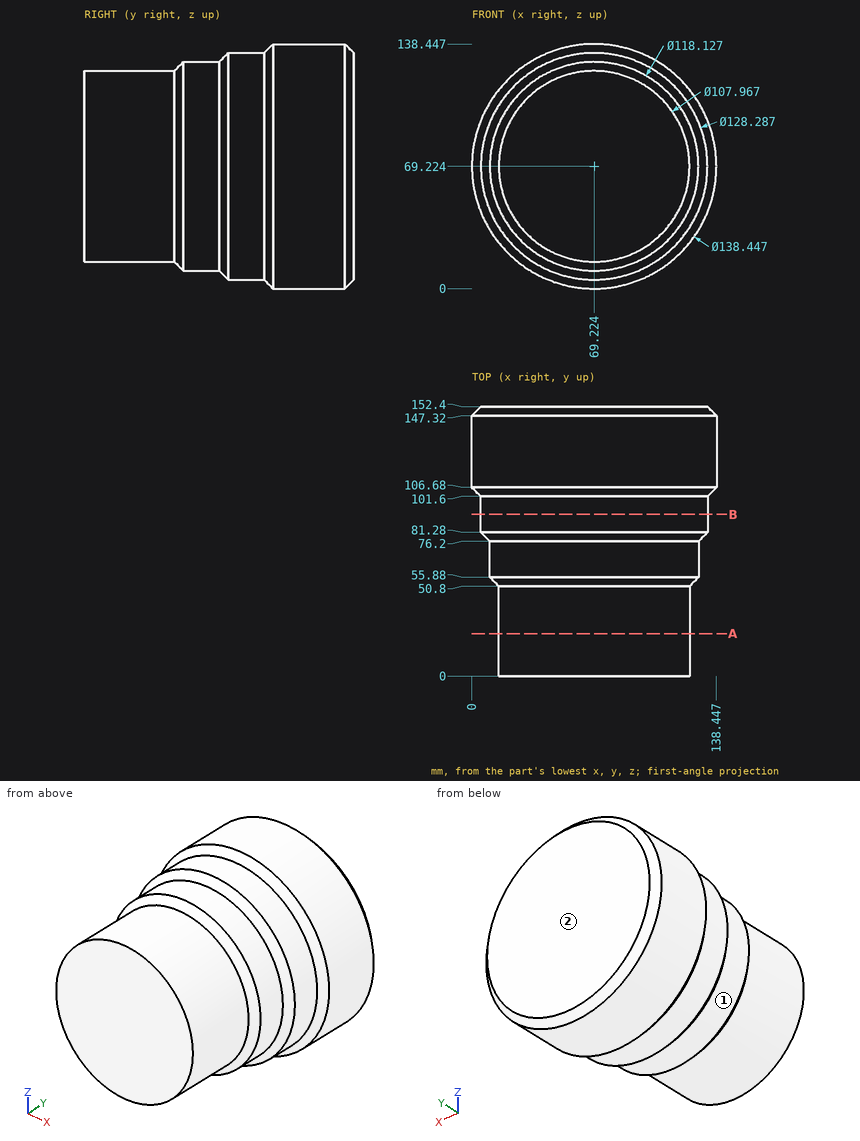
Geometry check sheet. Reference: drawing and pictorial views, mm from the part's lowest x, y, z. A direction names the side the tool comes from. Coordinates: 2 decimals unless noted, no trailing zeros. Write each loop counter-clockwise with the first axis right and the second up, starting at its lowest first coordinate (ties: lowest second). Pieces come first, ordered by that corner, then holes.
Item 1: Depth check by flat-ended pin: pin 1 Ø4 at (x, y) = (53.5, 72.5) entering from -Z; pin 2 Ø8 at (x, z) = (94, 88.5) entering from -Y; pin 3 Ø1 at (y, z) = (36, 68.5) entering from -X; pin 4 Ø4 at (y, z) = (36, 42.5) entering from -X (1 decimal). Enter the tip coordinate at first touch or a pass-through.
Numbers:
pin 1: stops at z = 11.78
pin 2: stops at y = 0
pin 3: stops at x = 15.24
pin 4: stops at x = 21.2
Item 2: Scan lines: probe 1 along Z at (x, y) = (75, 145) (1 decimal); probe 2 along Z at (x, y) = (109.5, 83) (1 decimal); probe 3 along X at (y, z) = (96.5, 55). Record each from-to range of solid material in increasing order.
Numbers:
probe 1: z = 0.2 to 138.2
probe 2: z = 19.3 to 119.1
probe 3: x = 6.68 to 131.77
Item 3: Cross-section at B-B on y = 91.5. Record the boundary of the cut face in (x, z).
Numbers:
outline: circle Ø128.29 at (69.22, 69.22)
Item 4: Access from +Z, -Z, +X, -X, +Y, -Y to the whole of each face (thin tool, end or side, straight path). Record for the marked faces 1 and 2.
Numbers:
face 1: -Y
face 2: +Z, -Z, +X, -X, +Y
Item 5: Cross-section at A-A on y = 24. Record the boundary of the cut face in (x, z), then the cut area to 3 significant figures.
Numbers:
outline: circle Ø107.97 at (69.22, 69.22)
area: 9,160 mm2
